```python
from build123d import *

# Parameters (mm, degrees)
F0_W     = 105
F0_H     = 15
F0_W_2   = 92.5
F0_H_2   = 5.6
F0_W_3   = 90
F0_H_3   = 3.1
F0_W_4   = 40
F1_DEPTH = 10
F2_DEPTH = 6.5
F3_W     = 13
F3_H     = 10
F4_DEPTH = 6
F5_D     = 8.1
F5_DEPTH = 22
F5_START = 6
F5_TIP   = 2.4334855071
F6_DEPTH = 4
F7_R     = 2.5
F8_R     = 1.5


with BuildPart() as f1:
    # F0 (on Top) → F1 (new body)
    with BuildSketch(Plane.XY):
        with Locations((72.5, 0)):
            Rectangle(F0_W, F0_H)
        with Locations((73.75, 0)):
            Rectangle(F0_W_2, F0_H_2, mode=Mode.SUBTRACT)
        with Locations((-72.5, 0)):
            Rectangle(F0_W, F0_H)
        with Locations((-73.75, 0)):
            Rectangle(F0_W_2, F0_H_2, mode=Mode.SUBTRACT)
        with Locations((-73.75, 0)):
            Rectangle(F0_W_2, F0_H_2)
        with Locations((-73.75, 0)):
            Rectangle(F0_W_3, F0_H_3, mode=Mode.SUBTRACT)
        with Locations((73.75, 0)):
            Rectangle(F0_W_2, F0_H_2)
        with Locations((73.75, 0)):
            Rectangle(F0_W_3, F0_H_3, mode=Mode.SUBTRACT)
        Rectangle(F0_W_4, F0_H)
    extrude(amount=F1_DEPTH)

    # F0 (on Top) → F2 (cut)
    with BuildSketch(Plane.XY):
        with Locations((73.75, 0)):
            Rectangle(F0_W_2, F0_H_2)
        with Locations((73.75, 0)):
            Rectangle(F0_W_3, F0_H_3, mode=Mode.SUBTRACT)
        with Locations((-73.75, 0)):
            Rectangle(F0_W_2, F0_H_2)
        with Locations((-73.75, 0)):
            Rectangle(F0_W_3, F0_H_3, mode=Mode.SUBTRACT)
    extrude(amount=F2_DEPTH, mode=Mode.SUBTRACT)

    # F3 (on face) → F4 (cut)
    with BuildSketch(Plane(origin=(0, 7.5, 0), x_dir=(-1, 0, 0), z_dir=(0, 1, 0))):
        with Locations((0, 5)):
            Rectangle(F3_W, F3_H)
    extrude(amount=-F4_DEPTH, mode=Mode.SUBTRACT)

    # F5
    # its depths count from where the whole tool has entered the part; down to there all is cleared
    with Locations(Plane(origin=(0, 7.5, 0), x_dir=(-1, 0, 0), z_dir=(0, 1, 0)).offset(-F5_START)):
        with Locations((0, 5)):
            Hole(F5_D / 2, depth=F5_DEPTH)
            with Locations((0, 0, -(F5_DEPTH + F5_TIP / 2))):  # 118° drill point
                Cone(0, F5_D / 2, F5_TIP, mode=Mode.SUBTRACT)

    # F0 (on Top) → F6 (cut)
    with BuildSketch(Plane.XY):
        with Locations((-72.5, 0)):
            Rectangle(F0_W, F0_H)
        with Locations((-73.75, 0)):
            Rectangle(F0_W_2, F0_H_2, mode=Mode.SUBTRACT)
        with Locations((72.5, 0)):
            Rectangle(F0_W, F0_H)
        with Locations((73.75, 0)):
            Rectangle(F0_W_2, F0_H_2, mode=Mode.SUBTRACT)
    extrude(amount=F6_DEPTH, mode=Mode.SUBTRACT)

    # F7
    f7_edges = [f1.edges().sort_by_distance(p)[0] for p in [
        (-27.5, 2.8, 5.25),
        (-27.5, -2.8, 5.25),
        (-120, 2.8, 5.25),
        (-120, -2.8, 5.25),
        (27.5, -2.8, 5.25),
        (120, -2.8, 5.25),
        (120, 2.8, 5.25),
        (27.5, 2.8, 5.25),
    ]]
    fillet(f7_edges, radius=F7_R)

    # F8
    f8_edges = [f1.edges().sort_by_distance(p)[0] for p in [
        (28.75, 1.55, 8.25),
        (28.75, -1.55, 8.25),
        (118.75, 1.55, 8.25),
        (118.75, -1.55, 8.25),
        (-28.75, -1.55, 8.25),
        (-28.75, 1.55, 8.25),
        (-118.75, 1.55, 8.25),
        (-118.75, -1.55, 8.25),
    ]]
    fillet(f8_edges, radius=F8_R)


solid = f1.part
```
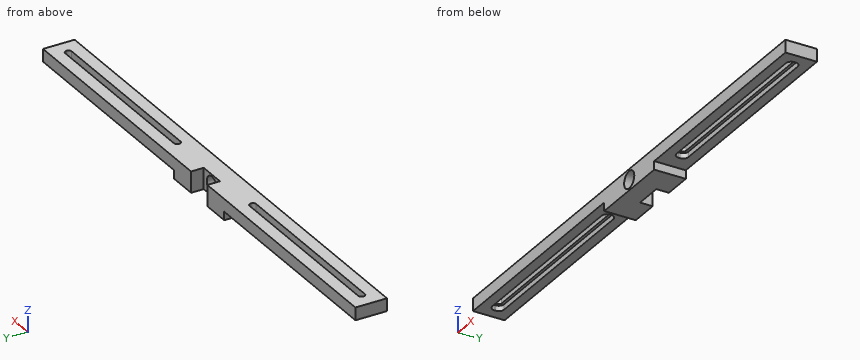
Verification items for the finished model (mm, model axes). Coordinates: 2 decimals unless noted, no trailing zeros. Loops run counter-clockwise (first coordinate to the right, second up) from the corner with the lowest first, then second, coordinate; pieces in that order, holes last. Notation, with made-up numbers: (47, 76.25) - (87, 76.25) arc R21 ccw to (87, 99.25) - close; hole circle Ø10 at (36, -30). An arc over 180 degrees is marked (long way). Answer as a JSON object with one key per item and string values.
(1) Scan lines: line 1 along Y through (x, z) = (49, 4.75); line 2 along Z through (x, y) = (0, -2); line 3 along Y through (x, z) = (-36, 6.75). Record each from-to range of solid material in increasing order.
Response:
{"line 1": "y = -7.5 to -2.8, 2.8 to 7.5", "line 2": "z = 0 to 0.95, 9.05 to 10", "line 3": "y = -7.5 to -1.55, 1.55 to 7.5"}
(2) Go/stop test with flat-tipped pins: pin 1 Ø4 at (x, y) = (-84.5, 3.5) entering from -Z; pin 2 Ø4.5 at (x, y) = (-56.5, 0) entering from -Z. Record where each tip stops, or that it passes through.
Response:
{"pin 1": "stops at z = 4", "pin 2": "stops at z = 6.5"}
(3) Cross-section at B-B, the plane x = -70. Record the boundary of the cut face in (y, z), then the cut area to 4 significant figures.
Response:
{"outline": "(-7.5, 4) - (-2.8, 4) - (-2.8, 6.5) - (-1.55, 6.5) - (-1.55, 10) - (-7.5, 10) - close; (1.55, 6.5) - (2.8, 6.5) - (2.8, 4) - (7.5, 4) - (7.5, 10) - (1.55, 10) - close", "area": "65.15 mm²"}
(4) Cross-section at A-A, the plane x = 0. Record the boundary of the cut face in (y, z), then the cut area to 3 significant figures.
Response:
{"outline": "(-7.5, 0) - (1.5, 0) - (1.5, 0.95) - (-7.5, 0.95) - close; (-7.5, 9.05) - (1.5, 9.05) - (1.5, 10) - (-7.5, 10) - close", "area": "17.1 mm²"}
